Check sheet for the modelled part. Datum: model origin and axes. Units: mm. Face numbers are marked on the shaded views. A direction names the side the tool comes from. Round coordinates to 2 decimals unless told otherwise and drop trailing zeros. Write each loop counter-clockwise with the first axis right and the second up, starting at its lowest first coordinate (ties: lowest second). Pieces come first, ordered by that corner, then holes.
from build123d import *
from build123d.topology import SkipClean

# Parameters (mm, degrees)
SKETCH1_R           = 15
BOSS_EXTRUDE1_DEPTH = 10.5
SKETCH2_R           = 11
CUT_EXTRUDE1_DEPTH  = 1
SKETCH3_R           = 12
SKETCH3_R_2         = 2.5
SKETCH3_R_3         = 1
CUT_EXTRUDE2_DEPTH  = 6
SKETCH3_4_R         = 2.5
SKETCH3_4_R_2       = 1
BOSS_EXTRUDE2_DEPTH = 2.5
FILLET1_R           = 1
CUT_EXTRUDE3_DEPTH  = 25.372115214


with BuildPart() as part:
    # Sketch1 → Boss-Extrude1 (new body)
    with BuildSketch(Plane.XY):
        with Locations(Location((0, 0, 0), (0, 0, 180))):
            Circle(SKETCH1_R)
    extrude(amount=BOSS_EXTRUDE1_DEPTH)

    # Sketch2 → Cut-Extrude1 (cut)
    with BuildSketch(Plane.XY.offset(10.5)):
        Circle(SKETCH2_R)
    extrude(amount=-CUT_EXTRUDE1_DEPTH, mode=Mode.SUBTRACT)

    # Sketch3 → Cut-Extrude2 (cut)
    with BuildSketch(Plane(origin=(0, 0, 0), x_dir=(-1, 0, 0), z_dir=(0, 0, -1))):
        Circle(SKETCH3_R)
        Circle(SKETCH3_R_2, mode=Mode.SUBTRACT)
        Circle(SKETCH3_R_3)
    extrude(amount=-CUT_EXTRUDE2_DEPTH, mode=Mode.SUBTRACT)

    # Sketch3_4 → Boss-Extrude2 (add)
    with BuildSketch(Plane(origin=(0, 0, 0), x_dir=(-1, 0, 0), z_dir=(0, 0, -1))):
        Circle(SKETCH3_4_R)
        Circle(SKETCH3_4_R_2, mode=Mode.SUBTRACT)
    extrude(amount=BOSS_EXTRUDE2_DEPTH)

    # Fillet1
    fillet1_edges = [part.edges().sort_by_distance(p)[0] for p in [
        (15, 0, 0),
        (15, 0, 10.5),
    ]]
    fillet(fillet1_edges, radius=FILLET1_R)

    # Sketch4 → Cut-Extrude3 (cut, through all)
    with SkipClean():  # the faces are left unmerged after this step: merging them gives an invalid solid
        with BuildSketch(Plane.XY.offset(9.5)):
            with BuildLine():
                Line((0, 2.5), (0, 9.339610027))
                ThreePointArc((0, 9.339610027), (2.417268949, 9.021370532), (4.669805013, 8.088339545))
                Line((4.669805013, 8.088339545), (1.25, 2.165063509))
                ThreePointArc((1.25, 2.165063509), (0.647047613, 2.414814566), (0, 2.5))
            make_face()
            with BuildLine():
                Line((2.377641291, 0.772542486), (8.882496976, 2.886098219))
                ThreePointArc((8.882496976, 2.886098219), (9.326810416, 0.488797422), (9.135517139, -1.941814112))
                Line((9.135517139, -1.941814112), (2.445369002, -0.519779227))
                ThreePointArc((2.445369002, -0.519779227), (2.496573837, 0.130839891), (2.377641291, 0.772542486))
            make_face()
            with BuildLine():
                Line((1.469463131, -2.022542486), (5.489685036, -7.555903232))
                ThreePointArc((5.489685036, -7.555903232), (3.347016895, -8.719277112), (0.976255084, -9.288446666))
                Line((0.976255084, -9.288446666), (0.261321158, -2.486304738))
                ThreePointArc((0.261321158, -2.486304738), (0.895919874, -2.333951066), (1.469463131, -2.022542486))
            make_face()
            with BuildLine():
                Line((-1.469463131, -2.022542486), (-5.489685036, -7.555903232))
                ThreePointArc((-5.489685036, -7.555903232), (-7.258240214, -5.877607034), (-8.532158316, -3.79876163))
                Line((-8.532158316, -3.79876163), (-2.283863644, -1.016841608))
                ThreePointArc((-2.283863644, -1.016841608), (-1.942864904, -1.573300978), (-1.469463131, -2.022542486))
            make_face()
            with BuildLine():
                Line((-2.377641291, 0.772542486), (-8.882496976, 2.886098219))
                ThreePointArc((-8.882496976, 2.886098219), (-7.832856045, 5.086716192), (-6.24941892, 6.940682863))
                Line((-6.24941892, 6.940682863), (-1.672826516, 1.857862064))
                ThreePointArc((-1.672826516, 1.857862064), (-2.09667642, 1.361597588), (-2.377641291, 0.772542486))
            make_face()
        extrude(amount=-CUT_EXTRUDE3_DEPTH, mode=Mode.SUBTRACT)


solid = part.part
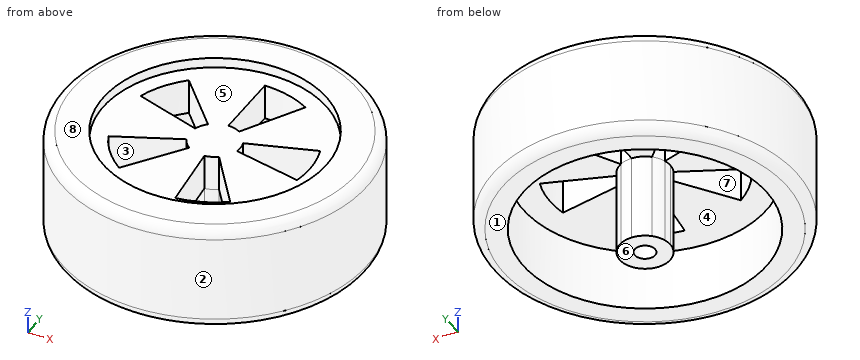
1. Go/stop test with flat-tipped pins: pin 1 (1.8 mm diameter, centred on y = 4.5, z = 8, fed in from +X); pin 2 (6 mm diameter, centred on y = 5, z = 0.5, fed in from +X); pin 3 (1 mm diameter, centred on x = -12, z = 0.5, fed in from +Y). Record where each tip stops, or that it passes through.
2. Sectioned sample at A-A, the plane z = 5. Enter the section's corners in (x, y), plus the area to 3 significant figures.
3. Sectioned sample at B-B, the plane z = 8. Enter the section's corners in (x, y).
4. Sectioned sample at C-C, the plane y = -1.5. Give the number of separate pieces and of enclosed holes in the cut face, plus the area to 3 significant figures.
5. Set-up check for the marked faces 4, 5, 6, 7 and 8: record each of +Z, -Z, +X, -X, +Y, -Y from which the full face is reachable in a straight line by a thin tool's end or side.
6. Release check for a two-part mould opening along Y. For the marked faces 1, 2 and 3 record: released by +Y, released by -Y, zero draft, split by the parting line, or undercut.
7. Scan lines: line 1 along X through (y, z) = (-4.5, 8.75); line 2 along Z through (x, y) = (5, 5.75); line 3 along Z through (x, y) = (-3, -12.5). Record each from-to range of solid material in increasing order.
Computed values:
1. pin 1: stops at x = 14.56
1. pin 2: stops at x = 14.86
1. pin 3: stops at y = 9.51
2. outline: circle Ø30 at (0, 0); circle Ø5 at (0, 0); hole circle Ø24 at (0, 0); hole circle Ø2 at (0, 0)
2. area: 271 mm2
3. outline: circle Ø30 at (0, 0); hole (-8.88, 2.89) - (-2.38, 0.77) arc R2.5 cw to (-1.67, 1.86) - (-6.25, 6.94) arc R9.34 ccw to start; hole (-8.53, -3.8) arc R9.34 ccw to (-5.49, -7.56) - (-1.47, -2.02) arc R2.5 cw to (-2.28, -1.02) - close; hole (0, 2.5) arc R2.5 cw to (1.25, 2.17) - (4.67, 8.09) arc R9.34 ccw to (0, 9.34) - close; hole (0.26, -2.49) - (0.98, -9.29) arc R9.34 ccw to (5.49, -7.56) - (1.47, -2.02) arc R2.5 cw to start; hole (2.38, 0.77) arc R2.5 cw to (2.45, -0.52) - (9.14, -1.94) arc R9.34 ccw to (8.88, 2.89) - close
4. separate pieces: 3
4. enclosed holes: 0
4. area: 170 mm2
5. face 4: -Z
5. face 5: +Z
5. face 6: -Z, +X, -X, +Y, -Y
5. face 7: +Z, -Z
5. face 8: +Z, +X, -X, +Y, -Y
6. face 1: zero draft
6. face 2: split by the parting line
6. face 3: undercut
7. line 1: x = -14.31 to -8.18, -3.27 to 0.47, 3.27 to 14.31
7. line 2: z = 6 to 9.5
7. line 3: z = 0 to 10.5
